Geometry: final body of the model. Coordinates: model frame, mm. Round coordinates to 2 decimals unless told otherwise and drop trailing zeros. Write each loop counter-clockwise with the first axis right and the second up, starting at its lowest first coordinate (ties: lowest second). Pieces come first, ordered by that corner, then holes. Notation, with made-up numbers: M -38,42 L -13,42 A19 cw -13,70 Z; hole C 38,7.5 d3. An arc over 180 degrees is marked long. Answer as CSV lines item,"result". Start each with the question number.
Q1. Mould query, pull axis Y, two halves, no side actions, for faces 1 (the flat face through (5, -2, 0)), 2 (the cylindrical face through (0.041, 4.496, 6.599)). Classes: pulls with the +Y half, pulls with the -Y half, needs draft (parallel to the pull), parting line crosses it, or undercut.
Q2. Section query A-A on z = 4.5. Output: boundary loops of the cut face in (x, y) (3 decimals).
Q3. First-contact query: pin 1 (12 mm diameter, centred on x = 4, y = 5, fed in from +Z); pin 2 (4 mm diameter, centred on x = -1, z = 2.5, fed in from -Y); pin 3 (5 mm diameter, centred on x = 1, y = -1, fed in from -Z). Flat tips, straight axial feed; report the tip coordinate or a pass-through.
Q4. Section query D-D on z = 2.75. Output: boundary loops of the cut face in (x, y) (3 decimals).
Q5. Ray query, probe 1 along X at (y, z) = (2.75, 6.75); probe 2 along Y at (x, z) = (-0.25, 1.25); probe 3 along X at (y, z) = (-3.5, 7). Return the intervals inside material, ascending.
```python
from build123d import *

# Parameters (mm, degrees)
F4_DEPTH = 7.2
F5_R     = 2


with BuildPart() as f2:
    # F1 (on Front) → F2 (revolve)
    with BuildSketch(Plane.XZ):
        with BuildLine():
            ThreePointArc((0, 9.9490633183), (-7.0530819666, 7.0381248849), (-10, 0))
            Line((-10, 0), (0, 0))
            Line((0, 0), (0, 9.9490633183))
        make_face()
    revolve(axis=Axis((0, 0, 4.9745316591), (0, 0, 1)))

    # F3 (on face) → F4 (cut)
    with BuildSketch(Plane(origin=(0, 0, 0), x_dir=(1, 0, 0), z_dir=(0, 0, -1))):
        Polygon((2.925, 5.0662486121), (-2.925, 5.0662486121), (-5.85, 0), (-2.925, -5.0662486121), (2.925, -5.0662486121), (5.85, 0), align=None)
    extrude(amount=-F4_DEPTH, mode=Mode.SUBTRACT)

    # F5
    f5_edges = [f2.edges().sort_by_distance(p)[0] for p in [
        (0, -5.066249, 7.2),
        (-4.3875, -2.533124, 7.2),
        (4.3875, -2.533124, 7.2),
        (4.3875, 2.533124, 7.2),
        (-4.3875, 2.533124, 7.2),
        (0, 5.066249, 7.2),
    ]]
    fillet(f5_edges, radius=F5_R)


solid = f2.part
```
Entries:
1,face 1,"needs draft"
1,face 2,"undercut"
2,outline,"C 0,0 d17.809; hole M -5.85,0 L -2.925,-5.066 L 2.925,-5.066 L 5.85,0 L 2.925,5.066 L -2.925,5.066 Z"
3,pin 1,"stops at z = 9.94"
3,pin 2,"stops at y = -9.97"
3,pin 3,"stops at z = 7.03"
4,outline,"C 0,0 d19.2; hole M -5.85,0 L -2.925,-5.066 L 2.925,-5.066 L 5.85,0 L 2.925,5.066 L -2.925,5.066 Z"
5,probe 1,"x = -6.8 to -3.41, 3.41 to 6.8"
5,probe 2,"y = -9.91 to -5.07, 5.07 to 9.91"
5,probe 3,"x = -6.17 to -2.53, 2.53 to 6.17"
